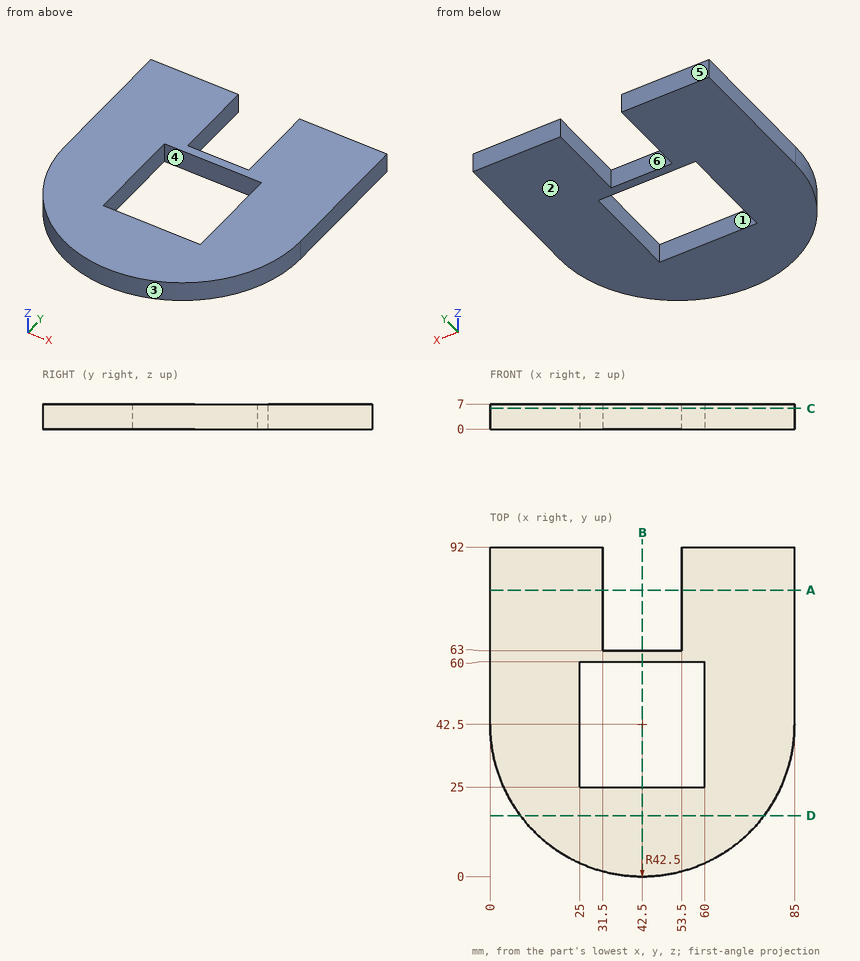
Check sheet for the drawn part. Datum: minimum x, y, z corner. Units: mm. A direction names the side the tool comes from. Round coordinates to 2 decimals unless told otherwise and drop trailing zeros. Order: outer loops, then holes, each group sorted by start corner. A loop starts at its lowest first (then second) coordinate and runs counter-clockwise, first axis right, second up. Notation, with made-up numbers: (-8.75, -5) -> (0.25, -5) arc R15 ccw to (0.25, 1) -> close; hole circle Ø4 at (-7.5, 80.25). An arc over 180 degrees is marked (long way). Put each result on its own line as item: value.
1) Section check B-B (x = 42.5). Record the cut outline in (y, z), then the cut area to 3 significant figures.
Final values:
outline: (0, 0) -> (25, 0) -> (25, 7) -> (0, 7) -> close; (60, 0) -> (63, 0) -> (63, 7) -> (60, 7) -> close
area: 196 mm^2
2) Set-up check for the marked faces 5 and 6: record each of +Z, -Z, +X, -X, +Y, -Y from which the full face is reachable in a straight line by a thin tool's end or side.
Final values:
face 5: +Z, -Z, +X, -X, +Y
face 6: +Z, -Z, +Y
3) Depth check by flat-ended pin: pin 1 (3.5 mm diameter, centred on x = 50, z = 4.5, fed in from +Y); pin 2 (2 mm diameter, centred on y = 13, z = 2.5, fed in from -X); pin 3 (2 mm diameter, centred on y = 39, z = 5, fed in from -X). Enter the tip coordinate at first touch or a pass-through.
Final values:
pin 1: stops at y = 63
pin 2: stops at x = 10.97
pin 3: stops at x = 0.07
4) Section check C-C (z = 5.75). Record the cut outline in (x, y).
Final values:
outline: (0, 42.5) arc R42.5 ccw to (85, 42.5) -> (85, 92) -> (53.5, 92) -> (53.5, 63) -> (31.5, 63) -> (31.5, 92) -> (0, 92) -> close; hole (25, 25) -> (60, 25) -> (60, 60) -> (25, 60) -> close
5) Mould release check, pull along X, two halves, no side actions. Record for the marked faces 1, 2, 3 and 4: +X half, -X half, draft (parallel to the pull), parting line (faces both ways), or undercut.
Final values:
face 1: undercut
face 2: draft
face 3: parting line
face 4: undercut
6) Section check D-D (y = 17). Record the cut outline in (x, z).
Final values:
outline: (8.5, 0) -> (76.5, 0) -> (76.5, 7) -> (8.5, 7) -> close
7) Material ranges on line 1 (X direction, y = 43.5, z = 6); line 2 (X direction, y = 86.5, z = 1.75); line 3 (Y direction, x = 40.5, z = 3.25), recorded low to high.
Final values:
line 1: x = 0 to 25, 60 to 85
line 2: x = 0 to 31.5, 53.5 to 85
line 3: y = 0.05 to 25, 60 to 63
8) Section check A-A (y = 80). Record the cut outline in (x, z).
Final values:
outline: (0, 0) -> (31.5, 0) -> (31.5, 7) -> (0, 7) -> close; (53.5, 0) -> (85, 0) -> (85, 7) -> (53.5, 7) -> close
